Can you work these out from the model? Positions are in its coordinate system, mm. Face numbers are marked on the shaded views. A direction names the side the tool comes from. Coordinates: 2 decimals unless noted, no trailing zeros. Order: outer loops, then holes, each group sorted by start corner. A loop starts at its lowest first (then second) coordinate and runs counter-clockwise, first axis right, second up. Notation, with made-up numbers: (31.5, 19) -> (71.5, 19) arc R20 cw to (71.5, 40) -> close; hole circle Ø3 at (-35.5, 6). An arc over 180 degrees is marked (long way). Answer in a Markdown table with one row per item. Add a question column.
1. If I drill on line 1 along Z through (x, y) = (-22, 11); line 2 along X through (y, z) = (2.5, 13.5); line 3 along Y through (x, z) = (22.5, 7), over which ranges is the centre line in solid material (lowest first)? Write a range as [from, to].
2. Imagine slicing it at C-C on z = 11. Write out the boundary of the cut face in (x, y).
3. Imagine slicing it at A-A on x = 0. Write out the boundary of the cut face in (y, z).
4. On a 3-axis mill with a long thin cutter (end or side, diameter ignored), from which of +Z, -Z, +X, -X, +Y, -Y can I reach the whole of each face in a straight line? I mean the marked faces 1 and 2. Say none if no direction works.
5. Will these pins go through, and if not, where does the flat tip stop? pin 1 (1.5 mm diameter, centred on x = 11, y = -22, fed in from +Z); pin 2 (6 mm diameter, centred on y = 1.5, z = 13, fed in from -X).
6. Imagine slicing it at D-D on z = 2.75. Write out the boundary of the cut face in (x, y).
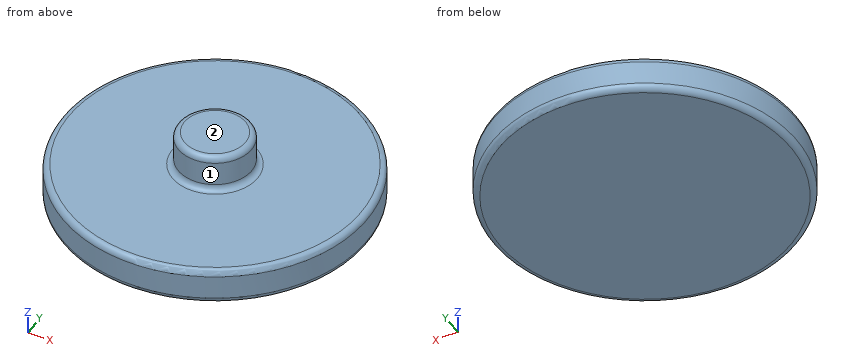
from build123d import *

# Parameters (mm, degrees)
F0_R     = 31.996319
F1_DEPTH = 7.62
F2_R     = 7.717623
F3_DEPTH = 7.62
F4_R     = 1.27


with BuildPart() as f1:
    # F0 (on Top) → F1 (new body)
    with BuildSketch(Plane.XY):
        Circle(F0_R)
    extrude(amount=F1_DEPTH)

    # F2 (on face) → F3 (join)
    with BuildSketch(Plane.XY.offset(7.62)):
        Circle(F2_R)
    extrude(amount=F3_DEPTH)

    # F4
    f4_edges = [f1.edges().sort_by_distance(p)[0] for p in [
        (-7.717623, 0, 15.24),
        (-31.996319, 0, 7.62),
        (-7.717623, 0, 7.62),
        (-31.996319, 0, 0),
    ]]
    fillet(f4_edges, radius=F4_R)


solid = f1.part
Answers follow:
| question | item | result |
|---|---|---|
| 1 | line 1 | z = [0, 7.62] |
| 1 | line 2 | x = [-7.3, 7.3] |
| 1 | line 3 | y = [-22.5, 22.5] |
| 2 | outline | circle Ø15.44 at (0, 0) |
| 3 | outline | (-32, 1.27) arc R1.27 ccw to (-30.73, 0) -> (30.73, 0) arc R1.27 ccw to (32, 1.27) -> (32, 6.35) arc R1.27 ccw to (30.73, 7.62) -> (8.99, 7.62) arc R1.27 cw to (7.72, 8.89) -> (7.72, 13.97) arc R1.27 ccw to (6.45, 15.24) -> (-6.45, 15.24) arc R1.27 ccw to (-7.72, 13.97) -> (-7.72, 8.89) arc R1.27 cw to (-8.99, 7.62) -> (-30.73, 7.62) arc R1.27 ccw to (-32, 6.35) -> close |
| 4 | face 1 | +Z |
| 4 | face 2 | +Z, +X, -X, +Y, -Y |
| 5 | pin 1 | stops at z = 7.62 |
| 5 | pin 2 | stops at x = -7.72 |
| 6 | outline | circle Ø63.99 at (0, 0) |
